from build123d import *

# Parameters (mm, degrees)
SKETCH053_R    = 11
SKETCH053_R_2  = 8
PAD_DEPTH      = 115
PAD_DEPTH_BACK = 7.5
SKETCH054_R    = 11
SKETCH054_R_2  = 3
PAD025_DEPTH   = 10
SKETCH055_R    = 7
SKETCH055_R_2  = 3
PAD026_DEPTH   = 45


with BuildPart() as part:
    # Sketch053 → Pad (new body, two sides)
    with BuildSketch(Plane.XZ) as pad_sk:
        Circle(SKETCH053_R)
        Circle(SKETCH053_R_2, mode=Mode.SUBTRACT)
    extrude(amount=-PAD_DEPTH)
    extrude(pad_sk.sketch, amount=PAD_DEPTH_BACK)

    # Sketch054 → Pad025 (join)
    with BuildSketch(Plane.XZ):
        Circle(SKETCH054_R)
        Circle(SKETCH054_R_2, mode=Mode.SUBTRACT)
    extrude(amount=-PAD025_DEPTH)

    # Sketch055 → Pad026 (join)
    with BuildSketch(Plane.XZ):
        Circle(SKETCH055_R)
        Circle(SKETCH055_R_2, mode=Mode.SUBTRACT)
    extrude(amount=PAD026_DEPTH)


solid = part.part
Work out the finished part from the listing and answer in its coordinate system (mm). A direction names the side the tool comes from. Round coordinates to 2 decimals unless told otherwise and drop trailing zeros. Write each loop counter-clockwise with the first axis right and the second up, starting at its lowest first coordinate (ties: lowest second). Pieces come first, ordered by that corner, then holes. Notation, with made-up numbers: (51.5, 79) -> (66.5, 79) arc R18 ccw to (66.5, 100) -> close; hole circle Ø6 at (-30, 70.25). An arc over 180 degrees is marked (long way). Write each question's results on one line, items separated by ' | '.
Item 1: Find the intervals of material crossed by line 1 along Z through (x, y) = (0, -4.25); line 2 along Z through (x, y) = (0, -31); line 3 along Y through (x, z) = (2, 9), in increasing order. Write a range as [from, to].
Result set:
line 1: [-11, -8], [-7, -3], [3, 7], [8, 11] | line 2: [-7, -3], [3, 7] | line 3: [-7.5, 115]
Item 2: Which of the six approach directions +Z, -Z, +X, -X, +Y, -Y give full straight-line access (tool end or side, diameter ignored) to faces 1 (the face through (-2, 115, -8)), 2 (the face through (-1.73, 61.76, -7.81)), 3 (the face through (6.466, -22.185, -2.681))?
Result set:
face 1: +Z, -Z, +X, -X, +Y | face 2: +Y | face 3: -Y
Item 3: Flat-ended cylindrical pins translate along their axes: P1, Ø6.5, axis at x = -1.5, z = 2, coming from the -Y side; P2, Ø13, axis at x = 0, z = 0, coming from the +Y side; P3, Ø8, axis at y = 78.5, z = 6.5, coming from the +X side; P4, Ø6, axis at x = -5, y = -3.5, coming from the -Z side. Find the tip coordinate at first contact, or state that the pin passes through.
Result set:
P1: y = -45 | P2: y = 10 | P3: x = 10.71 | P4: z = -10.82
Item 4: The mould has two halves that part along X. Classify faces 4 (the face through (-3, -17, 0)), 5 (the face through (1, -45, -3)), 6 (the face through (-2.38, 54.61, -10.74)): +X half, -X half, draft (parallel to the pull), parting line (faces both ways), or undercut.
Result set:
face 4: undercut | face 5: draft | face 6: parting line
Item 5: A cutting plane is placed at B-B, the plane z = 0. Determine the outline of the cut face in (x, y), plus the area to 4 significant figures.
Result set:
outline: (-11, -7.5) -> (-8, -7.5) -> (-8, 0) -> (-7, 0) -> (-7, -45) -> (-3, -45) -> (-3, 10) -> (-8, 10) -> (-8, 115) -> (-11, 115) -> close; (3, -45) -> (7, -45) -> (7, 0) -> (8, 0) -> (8, -7.5) -> (11, -7.5) -> (11, 115) -> (8, 115) -> (8, 10) -> (3, 10) -> close | area: 1,195 mm^2
Item 6: A cutting plane is placed at A-A, the plane x = 0. Determine the outline of the cut face in (y, z), plus the area to 4 significant figures.
Result set:
outline: (-45, -7) -> (0, -7) -> (0, -8) -> (-7.5, -8) -> (-7.5, -11) -> (115, -11) -> (115, -8) -> (10, -8) -> (10, -3) -> (-45, -3) -> close; (-45, 3) -> (10, 3) -> (10, 8) -> (115, 8) -> (115, 11) -> (-7.5, 11) -> (-7.5, 8) -> (0, 8) -> (0, 7) -> (-45, 7) -> close | area: 1,195 mm^2
Item 7: A cutting plane is placed at C-C, the plane y = 49. Determine the outline of the cut face in (x, z), plus the area to 3 significant figures.
Result set:
outline: circle Ø22 at (0, 0); hole circle Ø16 at (0, 0) | area: 179 mm^2
Item 8: A cutting plane is placed at D-D, the plane y = -9. Determine the outline of the cut face in (x, z), plus the area to 3 significant figures.
Result set:
outline: circle Ø14 at (0, 0); hole circle Ø6 at (0, 0) | area: 126 mm^2
